from build123d import *

# Parameters (mm, degrees)
SKETCH1_R           = 3.71
SKETCH1_R_2         = 1.925
BOSS_EXTRUDE1_DEPTH = 1.5875
FILLET1_R           = 2


with BuildPart() as part:
    # Sketch1 → Boss-Extrude1 (new body)
    with BuildSketch(Plane(origin=(0, 0, 0), x_dir=(1, 0, 0), z_dir=(0, 1, 0))):
        with BuildLine():
            Line((-53.793633628, 3.311040487), (-34.282911165, 27.071198303))
            ThreePointArc((-34.282911165, 27.071198303), (-33.620388047, 34.448624702), (-26.285908277, 33.413847594))
            Line((-26.285908277, 33.413847594), (-3.48495612, 44.647688368))
            ThreePointArc((-3.48495612, 44.647688368), (0, 49.02), (3.48495612, 44.647688368))
            Line((3.48495612, 44.647688368), (26.285908277, 33.413847594))
            ThreePointArc((26.285908277, 33.413847594), (33.620388047, 34.448624702), (34.282911165, 27.071198303))
            Line((34.282911165, 27.071198303), (53.793633628, 3.311040487))
            ThreePointArc((53.793633628, 3.311040487), (59.145, 0), (53.793633628, -3.311040487))
            Line((53.793633628, -3.311040487), (34.282911165, -27.071198303))
            ThreePointArc((34.282911165, -27.071198303), (33.620388047, -34.448624702), (26.285908277, -33.413847594))
            Line((26.285908277, -33.413847594), (3.48495612, -44.647688368))
            ThreePointArc((3.48495612, -44.647688368), (0, -49.02), (-3.48495612, -44.647688368))
            Line((-3.48495612, -44.647688368), (-26.285908277, -33.413847594))
            ThreePointArc((-26.285908277, -33.413847594), (-33.620388047, -34.448624702), (-34.282911165, -27.071198303))
            Line((-34.282911165, -27.071198303), (-53.793633628, -3.311040487))
            ThreePointArc((-53.793633628, -3.311040487), (-59.145, 0), (-53.793633628, 3.311040487))
        make_face()
        with Locations(Location((-30.445, 30.445, 0), (0, 0, 270))):
            Circle(SKETCH1_R, mode=Mode.SUBTRACT)
        with Locations(Location((0, -45.445, 0), (0, 0, 90))):
            Circle(SKETCH1_R_2, mode=Mode.SUBTRACT)
        with Locations(Location((-30.445, -30.445, 0), (0, 0, 90))):
            Circle(SKETCH1_R, mode=Mode.SUBTRACT)
        with Locations(Location((0, 45.445, 0), (0, 0, 270))):
            Circle(SKETCH1_R_2, mode=Mode.SUBTRACT)
        with Locations(Location((30.445, -30.445, 0), (0, 0, 270))):
            Circle(SKETCH1_R, mode=Mode.SUBTRACT)
        with Locations(Location((30.445, 30.445, 0), (0, 0, 90))):
            Circle(SKETCH1_R, mode=Mode.SUBTRACT)
        with BuildLine():
            Line((-52.518462907, 2.263930353), (-33.007740444, 26.024088169))
            ThreePointArc((-33.007740444, 26.024088169), (-27.269611953, 26.441375298), (-25.556672132, 31.933741299))
            Line((-25.556672132, 31.933741299), (-2.755719976, 43.167582073))
            ThreePointArc((-2.755719976, 43.167582073), (0, 41.87), (2.755719976, 43.167582073))
            Line((2.755719976, 43.167582073), (25.556672132, 31.933741299))
            ThreePointArc((25.556672132, 31.933741299), (27.269611953, 26.441375298), (33.007740444, 26.024088169))
            Line((33.007740444, 26.024088169), (52.518462907, 2.263930353))
            ThreePointArc((52.518462907, 2.263930353), (51.745, 0), (52.518462907, -2.263930353))
            Line((52.518462907, -2.263930353), (33.007740444, -26.024088169))
            ThreePointArc((33.007740444, -26.024088169), (27.269611953, -26.441375298), (25.556672132, -31.933741299))
            Line((25.556672132, -31.933741299), (2.755719976, -43.167582073))
            ThreePointArc((2.755719976, -43.167582073), (0, -41.87), (-2.755719976, -43.167582073))
            Line((-2.755719976, -43.167582073), (-25.556672132, -31.933741299))
            ThreePointArc((-25.556672132, -31.933741299), (-27.269611953, -26.441375298), (-33.007740444, -26.024088169))
            Line((-33.007740444, -26.024088169), (-52.518462907, -2.263930353))
            ThreePointArc((-52.518462907, -2.263930353), (-51.745, 0), (-52.518462907, 2.263930353))
        make_face(mode=Mode.SUBTRACT)
    extrude(amount=BOSS_EXTRUDE1_DEPTH)

    # Fillet1
    fillet1_edges = [part.edges().sort_by_distance(p)[0] for p in [
        (26.285908277, 0.79375, 33.413847594),
        (3.48495612, 0.79375, 44.647688368),
        (-3.48495612, 0.79375, 44.647688368),
        (-26.285908277, 0.79375, 33.413847594),
        (-34.282911165, 0.79375, 27.071198303),
        (-53.793633628, 0.79375, 3.311040487),
        (-53.793633628, 0.79375, -3.311040487),
        (-34.282911165, 0.79375, -27.071198303),
        (-26.285908277, 0.79375, -33.413847594),
        (-3.48495612, 0.79375, -44.647688368),
        (3.48495612, 0.79375, -44.647688368),
        (26.285908277, 0.79375, -33.413847594),
        (34.282911165, 0.79375, -27.071198303),
        (53.793633628, 0.79375, -3.311040487),
        (53.793633628, 0.79375, 3.311040487),
        (34.282911165, 0.79375, 27.071198303),
        (-52.518462907, 0.79375, -2.263930353),
        (-52.518462907, 0.79375, 2.263930353),
        (-33.007740444, 0.79375, 26.024088169),
        (-25.556672132, 0.79375, 31.933741299),
        (-2.755719976, 0.79375, 43.167582073),
        (2.755719976, 0.79375, 43.167582073),
        (25.556672132, 0.79375, 31.933741299),
        (33.007740444, 0.79375, 26.024088169),
        (52.518462907, 0.79375, 2.263930353),
        (52.518462907, 0.79375, -2.263930353),
        (33.007740444, 0.79375, -26.024088169),
        (25.556672132, 0.79375, -31.933741299),
        (2.755719976, 0.79375, -43.167582073),
        (-2.755719976, 0.79375, -43.167582073),
        (-25.556672132, 0.79375, -31.933741299),
        (-33.007740444, 0.79375, -26.024088169),
    ]]
    fillet(fillet1_edges, radius=FILLET1_R)


solid = part.part
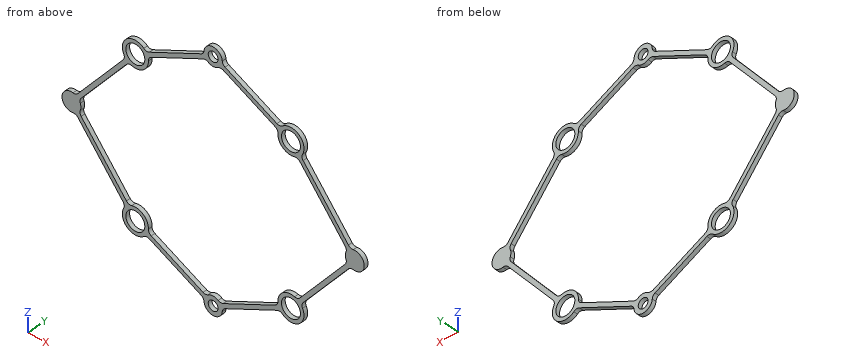
Verification items for the finished model (mm, model axes). Coordinates: 2 decimals unless noted, no trailing zeros. Write each loop counter-clockwise with the first axis right and the second up, starting at its lowest first coordinate (ties: lowest second). Pieces come first, ordered by that corner, then holes. Notation, with made-up numbers: M 38,3.5 L 75,3.5 A19 cw 75,19.5 Z; hole C -23.5,-37.75 d2. An arc over 180 degrees is marked long. One line per question, with ' | ' between items.
1) Material ranges on L1, parallel to X at y = 1.55, z = 28; L2, parallel to Z at x = 33.5, y = 1.35; L3, parallel to Z at x = -28, y = 0.8, recorded low to high.
Solutions:
L1: -34.94 to -33.24, -27.65 to -25.96, 25.96 to 27.65, 33.24 to 34.94 | L2: -34.54 to -32.55, -28.34 to -25.28, 25.28 to 28.34, 32.55 to 34.54 | L3: -34.93 to -33.24, -27.65 to -25.96, 25.96 to 27.65, 33.24 to 34.93
2) Sectioned sample at A-A on x = 0. Record the cut outline in (y, z).
Solutions:
outline: M 0,-49.02 L 1.59,-49.02 L 1.59,-47.37 L 0,-47.37 Z; M 0,-43.52 L 1.59,-43.52 L 1.59,-41.87 L 0,-41.87 Z; M 0,41.87 L 1.59,41.87 L 1.59,43.52 L 0,43.52 Z; M 0,47.37 L 1.59,47.37 L 1.59,49.02 L 0,49.02 Z
3) Sectioned sample at C-C on x = -48. Record the cut outline in (y, z), then the cut area to 3 significant figures.
Solutions:
outline: M 0,-10.37 L 1.59,-10.37 L 1.59,-7.77 L 0,-7.77 Z; M 0,7.77 L 1.59,7.77 L 1.59,10.37 L 0,10.37 Z | area: 8.26 mm^2
4) Depth check by flat-ended pin: pin 1 Ø6 at (x, z) = (-30.445, 30.445) entering from +Y. Enter the tip coordinate at first touch or a pass-through.
Solutions:
pin 1: through
5) Sectioned sample at D-D on y = 1. State how many separate pieces and enclosed holes the cut face has, then the cut area to 3 significant figures.
Solutions:
separate pieces: 1 | enclosed holes: 7 | area: 678 mm^2
6) Sectioned sample at B-B on z = 0. Record the cut outline in (x, y) (1 decimal).
Solutions:
outline: M -59.1,0 L -51.7,0 L -51.7,1.6 L -59.1,1.6 Z; M 51.7,0 L 59.1,0 L 59.1,1.6 L 51.7,1.6 Z
